```python
from build123d import *

# Parameters (mm, degrees)
SKETCH_1_R      = 10.5
SKETCH_1_R_2    = 4.5
EXTRUDE_1_DEPTH = 2
SKETCH_2_R      = 10.5
SKETCH_2_R_2    = 7.525
EXTRUDE_2_DEPTH = 15
EXTRUDE_START   = 15
SKETCH_3_R      = 10.5
SKETCH_3_R_2    = 7.525
EXTRUDE_3_DEPTH = 15


with BuildPart() as part:
    # 草图1 → 凸台-拉伸1 (new body)
    with BuildSketch(Plane.XY):
        Circle(SKETCH_1_R)
        Circle(SKETCH_1_R_2, mode=Mode.SUBTRACT)
    extrude(amount=EXTRUDE_1_DEPTH)

    # 草图2 → 凸台-拉伸2 (add)
    with BuildSketch(Plane.XY.offset(2)):
        Circle(SKETCH_2_R)
        Circle(SKETCH_2_R_2, mode=Mode.SUBTRACT)
    extrude(amount=EXTRUDE_2_DEPTH)

    # 草图3 → 凸台-拉伸3 (add)
    with BuildSketch(Plane(origin=(0, 0, 0), x_dir=(-1, 0, 0), z_dir=(0, 0, -1)).offset(EXTRUDE_START)):
        Circle(SKETCH_3_R)
        with Locations(Location((0, 0, 0), (0, 0, 180))):
            Circle(SKETCH_3_R_2, mode=Mode.SUBTRACT)
    extrude(amount=-EXTRUDE_3_DEPTH)


solid = part.part
```
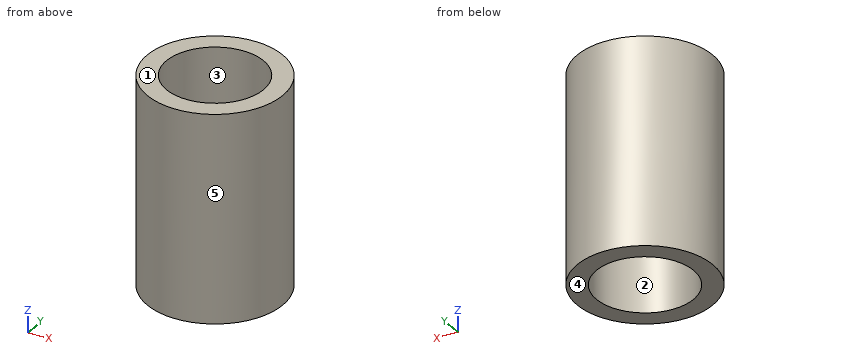
Geometry: final body of the model. Coordinates: model frame, mm. Face numbers are marked on the shaded views. A direction names the side the tool comes from. Round coordinates to 2 decimals unless told otherwise and drop trailing zeros. Order: outer loops, then holes, each group sorted by start corner. A loop starts at its lowest first (then second) coordinate and runs counter-clockwise, first axis right, second up. Notation, with made-up numbers: (29.25, 85.25) -> (73.25, 85.25) arc R31 cw to (73.25, 123.25) -> close; hole circle Ø9 at (-11, -11.75). An arc over 180 degrees is marked (long way). Use one line per item in the form item = value.
(1) Access query for the marked faces 1 and 2. Directions: +Z, -Z, +X, -X, +Y, -Y. A direction counts if a zero-diameter tool reaches every point of the face in a straight line with its end or side. Return the directions, or none.
Results list:
face_1 = +Z, +X, -X, +Y, -Y
face_2 = -Z
(2) Draft query along X for the marked faces 3, 4 and 5. Return one class per face: pulls with the +X half, pulls with the -X half, needs draft (parallel to the pull), parting line crosses it, or undercut.
Results list:
face_3 = undercut
face_4 = needs draft
face_5 = parting line crosses it
(3) Section A-A on x = 0. Return loops of the section in (y, z) (3 decimals).
Results list:
outline = (-10.5, -15) -> (-7.525, -15) -> (-7.525, 0) -> (-4.5, 0) -> (-4.5, 2) -> (-7.525, 2) -> (-7.525, 17) -> (-10.5, 17) -> close; (4.5, 0) -> (7.525, 0) -> (7.525, -15) -> (10.5, -15) -> (10.5, 17) -> (7.525, 17) -> (7.525, 2) -> (4.5, 2) -> close
(4) Ray query, probe 1 along Y at (x, z) = (0, 0.85); probe 2 along Y at (x, z) = (0, -5.25) (3 decimals); probe 3 along Z at (x, y) = (4.5, -3.25). Return the intervals inside material, ascending. Write a range as [from, to].
Results list:
probe_1 = [-10.5, -4.5], [4.5, 10.5]
probe_2 = [-10.5, -7.525], [7.525, 10.5]
probe_3 = [0, 2]
(5) Section C-C on z = -12.5. Return loops of the section in (x, y) (3 decimals), and give its area (3 significant figures).
Results list:
outline = circle Ø21 at (0, 0); hole circle Ø15.05 at (0, 0)
area = 168 mm^2
(6) Section D-D on y = 6.75. Return loops of the section in (x, z).
Results list:
outline = (-8.04, -15) -> (-3.33, -15) -> (-3.33, 0) -> (3.33, 0) -> (3.33, -15) -> (8.04, -15) -> (8.04, 17) -> (3.33, 17) -> (3.33, 2) -> (-3.33, 2) -> (-3.33, 17) -> (-8.04, 17) -> close
(7) First-contact query: pin 1 Ø7.5 at (x, y) = (1.5, -2.5) entering from -Z; pin 2 Ø3 at (y, z) = (5, 8) entering from +X; pin 3 Ø3 at (y, z) = (4.5, 11) entering from -X. Flat tips, straight axial feed; report the tip coordinate or a pass-through.
Results list:
pin_1 = 0
pin_2 = 9.9
pin_3 = -10.06
